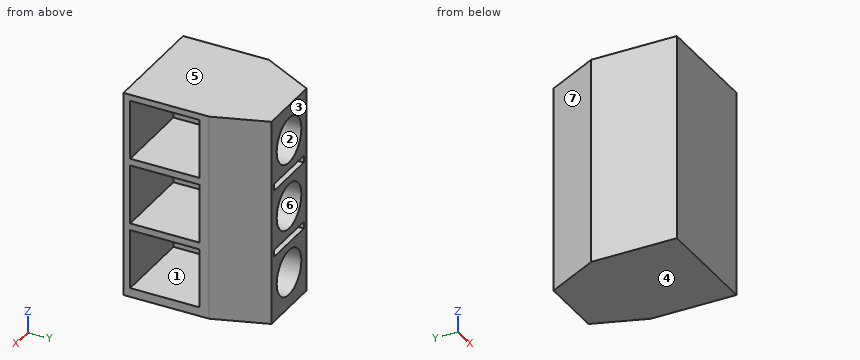
from build123d import *

# Parameters (mm, degrees)
BOSS_EXTRUDE1_DEPTH = 15
SKETCH2_W           = 4
SKETCH2_H           = 0.5
SKETCH2_R           = 1.65
CUT_EXTRUDE1_DEPTH  = 9.2
SKETCH3_W           = 4.3
SKETCH3_H           = 5
CUT_EXTRUDE2_DEPTH  = 5.8


with BuildPart() as part:
    # Sketch1 → Boss-Extrude1 (new body)
    with BuildSketch(Plane.XY):
        Polygon((-363.835743374, 0), (-355.835743374, 0), (-355.835743374, 6.2), (-357.144738603, 10), (-361.844738603, 10), (-363.835743374, 6.2), align=None)
    extrude(amount=BOSS_EXTRUDE1_DEPTH)

    # Sketch2 → Cut-Extrude1 (cut)
    with BuildSketch(Plane(origin=(0, 10, 0), x_dir=(1, 0, 0), z_dir=(0, 1, 0))):
        with Locations((-359.47498497, -5.05)):
            Rectangle(SKETCH2_W, SKETCH2_H)
        with Locations((-359.47498497, -9.95)):
            Rectangle(SKETCH2_W, SKETCH2_H)
        with Locations((-359.494738603, -2.6)):
            Circle(SKETCH2_R)
        with Locations((-359.494738603, -7.5)):
            Circle(SKETCH2_R)
        with Locations((-359.494738603, -12.4)):
            Circle(SKETCH2_R)
    extrude(amount=-CUT_EXTRUDE1_DEPTH, mode=Mode.SUBTRACT)

    # Sketch3 → Cut-Extrude2 (cut)
    with BuildSketch(Plane(origin=(-355.835743374, 0, 0), x_dir=(0, 0, -1), z_dir=(1, 0, 0))):
        with Locations((-12.4, 2.989005182)):
            Rectangle(SKETCH3_W, SKETCH3_H)
        with Locations((-7.6, 2.989005182)):
            Rectangle(SKETCH3_W, SKETCH3_H)
        with Locations((-2.8, 2.989005182)):
            Rectangle(SKETCH3_W, SKETCH3_H)
    extrude(amount=-CUT_EXTRUDE2_DEPTH, mode=Mode.SUBTRACT)


solid = part.part
The listing builds one solid part. Answer for the finished solid, in the listing's coordinates (mm). Face numbers are marked on the shaded views. A direction names the side the tool comes from. Round coordinates to 2 decimals unless told otherwise and drop trailing zeros. Write each loop counter-clockwise with the first axis right and the second up, starting at its lowest first coordinate (ties: lowest second). Pieces come first, ordered by that corner, then holes. Notation, with made-up numbers: (24.5, 0) - (29.5, 0) arc R21 ccw to (29.5, 37) - close; hole circle Ø9 at (-15.5, 64.25). An arc over 180 degrees is marked (long way). Use a Markdown table: item, result. Add a question column.
1. Consider line 1 (Z direction, x = -358, y = 6.75); line 2 (Z direction, x = -357, y = 2.5); line 3 (Y direction, x = -357.5, z = 6.5). Determine where each line is inside the solid, lowest interval first.
2. The part is cut by section B-B (y = 4.75). Write down the section's boundary in (x, z).
3. The part is cut by section D-D (z = 12.75). Write down the section's boundary in (x, y), and give its area (3 significant figures).
4. A tool of negligible diameter and unlimited length cuts with its end or side. For the marked faces 1, 2 and 3, from which of +Z, -Z, +X, -X, +Y, -Y can it reach the whole face along a straight path? Write none if from no direction.
5. The part is cut by section A-A (z = 2.6). Write down the section's boundary in (x, y).
6. Flat-ended cylindrical pins translate along their axes: P1, Ø2, axis at y = 4, z = 6.5, coming from the +X side; P2, Ø2, axis at y = 9, z = 5, coming from the -X side. Find the tip coordinate at first contact, or state that the pin passes through.
7. For a pull along Z with two mould halves and no side action, classify the marked faces 4, 5, 6 and 7 as +Z half, -Z half, draft (parallel to the pull), parting line (faces both ways), or undercut.
8. The part is cut by section C-C (x = -359.5). Give the number of separate pieces and of enclosed holes in the cut face, and give its area (3 significant figures).
Reported:
| question | item | result |
|---|---|---|
| 1 | line 1 | 0 to 1.9, 3.3 to 4.8, 5.3 to 6.8, 8.2 to 9.7, 10.2 to 11.7, 13.1 to 15 |
| 1 | line 2 | 0 to 0.65, 4.95 to 5.45, 9.75 to 10.25, 14.55 to 15 |
| 1 | line 3 | 0 to 0.49, 5.49 to 10 |
| 2 | outline | (-363.84, 0) - (-355.84, 0) - (-355.84, 0.65) - (-361.64, 0.65) - (-361.64, 4.95) - (-361.47, 4.95) - (-361.47, 5.3) - (-357.47, 5.3) - (-357.47, 4.95) - (-355.84, 4.95) - (-355.84, 5.45) - (-361.64, 5.45) - (-361.64, 9.75) - (-361.47, 9.75) - (-361.47, 10.2) - (-357.47, 10.2) - (-357.47, 9.75) - (-355.84, 9.75) - (-355.84, 10.25) - (-361.64, 10.25) - (-361.64, 14.55) - (-355.84, 14.55) - (-355.84, 15) - (-363.84, 15) - close |
| 3 | outline | (-363.84, 0) - (-355.84, 0) - (-355.84, 0.49) - (-361.64, 0.49) - (-361.64, 5.49) - (-361.11, 5.49) - (-361.11, 10) - (-361.84, 10) - (-363.84, 6.2) - close; (-357.88, 5.49) - (-355.84, 5.49) - (-355.84, 6.2) - (-357.14, 10) - (-357.88, 10) - close |
| 3 | area | 30.2 mm^2 |
| 4 | face 1 | +X |
| 4 | face 2 | +Y |
| 4 | face 3 | +Z, -Z, +X, -X, +Y |
| 5 | outline | (-363.84, 0) - (-355.84, 0) - (-355.84, 0.49) - (-361.64, 0.49) - (-361.64, 5.49) - (-361.14, 5.49) - (-361.14, 10) - (-361.84, 10) - (-363.84, 6.2) - close; (-357.84, 5.49) - (-355.84, 5.49) - (-355.84, 6.2) - (-357.14, 10) - (-357.84, 10) - close |
| 6 | P1 | x = -361.64 |
| 6 | P2 | x = -362.89 |
| 7 | face 4 | -Z half |
| 7 | face 5 | +Z half |
| 7 | face 6 | undercut |
| 7 | face 7 | draft |
| 8 | separate pieces | 3 |
| 8 | enclosed holes | 0 |
| 8 | area | 32.6 mm^2 |
